Part model, mm, in its own coordinate system. Face numbers are marked on the shaded views. A direction names the side the tool comes from. Round coordinates to 2 decimals unless told otherwise and drop trailing zeros. Write each loop counter-clockwise with the first axis right and the second up, starting at its lowest first coordinate (ties: lowest second). Pieces come first, ordered by that corner, then holes. Notation, with made-up numbers: (74.25, -33.75) -> (118.25, -33.75) arc R19 ccw to (118.25, -9.75) -> close; hole circle Ø10 at (-12, 62.25). An arc over 180 degrees is marked (long way). Use CSV: the item, a comma, the result in double quotes. Start each with the question number.
(1) Drop flat-ended pins along their axis: pin 1 (6 mm diameter, centred on x = -36.5, y = 25.83, fed in from -Z); pin 2 (17.5 mm diameter, centred on y = 21, z = 88.5, fed in from +X); pin 3 (1.5 mm diameter, centred on x = -40.5, z = 2.5, fed in from +Y); pin 4 (19 mm diameter, centred on y = -11.5, z = 72.5, fed in from -X). Give the stop position or say it passes through.
(2) Saw through at C-C (y = 0). Give the cut face in (x, z).
(3) Which spindle directions (+Z, -Z, +X, -X, +Y, -Y) get a long thin tool onto all of the face, cutting with end or side? Do the marked faces 1 and 2. Say none if no direction does.
(4) Saw through at A-A (x = -48.5). Give the cut face in (y, z), plus the area to 3 significant figures.
(5) Two-plate mould, pull along Y, no slides. Class the marked faces 3, 4 and 5: released by +Y, released by -Y, zero draft, split by the parting line, or undercut.
(6) Probe line 1 (X direction, y = 17.5, z = 61.5); line 2 (Y direction, x = 2.5, z = 91.5); line 3 (X direction, y = 0, z = 104). List the from-to ranges inside material, lowest first. Write a range as [from, to].
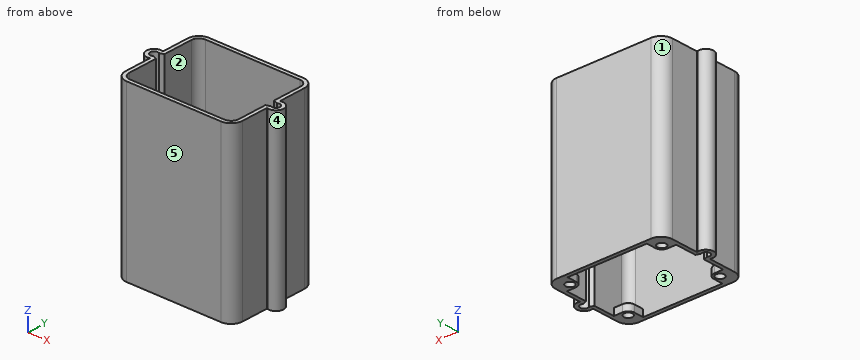
```python
from build123d import *

# Parameters (mm, degrees)
EXTRUDE_THIN1_DEPTH = 135
SKETCH6_R           = 3.429
BOSS_EXTRUDE1_DEPTH = 6
FILLET1_R           = 1


with BuildPart() as part:
    # Sketch4 → Extrude-Thin1 (new body)
    with BuildSketch(Plane.XY):
        with BuildLine():
            Line((-46.5, 27.5), (-46.5, 5.907156632))
            Line((-46.5, 5.907156632), (-46.877529279, 5.776468537))
            ThreePointArc((-46.877529279, 5.776468537), (-54.5, 0), (-46.877529279, -5.776468537))
            Line((-46.877529279, -5.776468537), (-46.5, -5.907156632))
            Line((-46.5, -5.907156632), (-46.5, -27.5))
            ThreePointArc((-46.5, -27.5), (-43.863961031, -33.863961031), (-37.5, -36.5))
            Line((-37.5, -36.5), (37.5, -36.5))
            ThreePointArc((37.5, -36.5), (43.863961031, -33.863961031), (46.5, -27.5))
            Line((46.5, -27.5), (46.5, -5.907156632))
            Line((46.5, -5.907156632), (46.877529279, -5.776468537))
            ThreePointArc((46.877529279, -5.776468537), (54.5, 0), (46.877529279, 5.776468537))
            Line((46.877529279, 5.776468537), (46.5, 5.907156632))
            Line((46.5, 5.907156632), (46.5, 27.5))
            ThreePointArc((46.5, 27.5), (43.863961031, 33.863961031), (37.5, 36.5))
            Line((37.5, 36.5), (-37.5, 36.5))
            ThreePointArc((-37.5, 36.5), (-43.863961031, 33.863961031), (-46.5, 27.5))
        make_face()
        with BuildLine():
            Line((-43.5, 27.5), (-43.5, 3.770994321))
            Line((-43.5, 3.770994321), (-46.9586126, 2.573737532))
            ThreePointArc((-46.9586126, 2.573737532), (-51.5, 0), (-46.9586126, -2.573737532))
            Line((-46.9586126, -2.573737532), (-43.5, -3.770994321))
            Line((-43.5, -3.770994321), (-43.5, -27.5))
            ThreePointArc((-43.5, -27.5), (-41.742640687, -31.742640687), (-37.5, -33.5))
            Line((-37.5, -33.5), (37.5, -33.5))
            ThreePointArc((37.5, -33.5), (41.742640687, -31.742640687), (43.5, -27.5))
            Line((43.5, -27.5), (43.5, -3.770994321))
            Line((43.5, -3.770994321), (46.9586126, -2.573737532))
            ThreePointArc((46.9586126, -2.573737532), (51.5, 0), (46.9586126, 2.573737532))
            Line((46.9586126, 2.573737532), (43.5, 3.770994321))
            Line((43.5, 3.770994321), (43.5, 27.5))
            ThreePointArc((43.5, 27.5), (41.742640687, 31.742640687), (37.5, 33.5))
            Line((37.5, 33.5), (-37.5, 33.5))
            ThreePointArc((-37.5, 33.5), (-41.742640687, 31.742640687), (-43.5, 27.5))
        make_face(mode=Mode.SUBTRACT)
    extrude(amount=EXTRUDE_THIN1_DEPTH)

    # Sketch6 → Boss-Extrude1 (add)
    with BuildSketch(Plane(origin=(0, 0, 0), x_dir=(-1, 0, 0), z_dir=(0, 0, -1))):
        with BuildLine():
            Line((-31.5, 25.830127019), (-31.5, 33.5))
            Line((-31.5, 33.5), (-37.5, 33.5))
            ThreePointArc((-37.5, 33.5), (-41.742640687, 31.742640687), (-43.5, 27.5))
            Line((-43.5, 27.5), (-43.5, 20.830127019))
            Line((-43.5, 20.830127019), (-36.5, 20.830127019))
            ThreePointArc((-36.5, 20.830127019), (-32.964466094, 22.294593113), (-31.5, 25.830127019))
        make_face()
        with Locations((-36.5, 25.830127019)):
            Circle(SKETCH6_R, mode=Mode.SUBTRACT)
        with BuildLine():
            Line((37.5, 33.5), (31.5, 33.5))
            Line((31.5, 33.5), (31.5, 25.830127019))
            ThreePointArc((31.5, 25.830127019), (32.964466094, 22.294593113), (36.5, 20.830127019))
            Line((36.5, 20.830127019), (43.5, 20.830127019))
            Line((43.5, 20.830127019), (43.5, 27.5))
            ThreePointArc((43.5, 27.5), (41.742640687, 31.742640687), (37.5, 33.5))
        make_face()
        with Locations((36.5, 25.830127019)):
            Circle(SKETCH6_R, mode=Mode.SUBTRACT)
        with BuildLine():
            Line((31.5, -25.830127019), (31.5, -33.5))
            Line((31.5, -33.5), (37.5, -33.5))
            ThreePointArc((37.5, -33.5), (41.742640687, -31.742640687), (43.5, -27.5))
            Line((43.5, -27.5), (43.5, -20.830127019))
            Line((43.5, -20.830127019), (36.5, -20.830127019))
            ThreePointArc((36.5, -20.830127019), (32.964466094, -22.294593113), (31.5, -25.830127019))
        make_face()
        with Locations((36.5, -25.830127019)):
            Circle(SKETCH6_R, mode=Mode.SUBTRACT)
        with BuildLine():
            Line((-37.5, -33.5), (-31.5, -33.5))
            Line((-31.5, -33.5), (-31.5, -25.830127019))
            ThreePointArc((-31.5, -25.830127019), (-32.964466094, -22.294593113), (-36.5, -20.830127019))
            Line((-36.5, -20.830127019), (-43.5, -20.830127019))
            Line((-43.5, -20.830127019), (-43.5, -27.5))
            ThreePointArc((-43.5, -27.5), (-41.742640687, -31.742640687), (-37.5, -33.5))
        make_face()
        with Locations((-36.5, -25.830127019)):
            Circle(SKETCH6_R, mode=Mode.SUBTRACT)
    extrude(amount=-BOSS_EXTRUDE1_DEPTH)

    # Fillet1
    fillet1_edges = [part.edges().sort_by_distance(p)[0] for p in [
        (-40, 20.830127019, 6),
        (-32.964466094, 22.294593113, 6),
        (-31.5, 29.665063509, 6),
        (-32.964466094, -22.294593113, 6),
        (-40, -20.830127019, 6),
        (-31.5, -29.665063509, 6),
        (40, -20.830127019, 6),
        (32.964466094, -22.294593113, 6),
        (31.5, -29.665063509, 6),
        (32.964466094, 22.294593113, 6),
        (40, 20.830127019, 6),
        (31.5, 29.665063509, 6),
    ]]
    fillet(fillet1_edges, radius=FILLET1_R)


solid = part.part
```
Answers:
1,pin 1,"passes through"
1,pin 2,"stops at x = 46.5"
1,pin 3,"stops at y = 36.21"
1,pin 4,"stops at x = -54.16"
2,outline,"(-54.5, 0) -> (-51.5, 0) -> (-51.5, 135) -> (-54.5, 135) -> close; (51.5, 0) -> (54.5, 0) -> (54.5, 135) -> (51.5, 135) -> close"
3,face 1,"+Z, -Z, -X, +Y"
3,face 2,"+Z"
4,outline,"(-6, 0) -> (-3, 0) -> (-3, 135) -> (-6, 135) -> close; (3, 0) -> (6, 0) -> (6, 135) -> (3, 135) -> close"
4,area,"810 mm²"
5,face 3,"undercut"
5,face 4,"split by the parting line"
5,face 5,"released by -Y"
6,line 1,"x = [-46.5, -43.5], [43.5, 46.5]"
6,line 2,"y = [-36.5, -33.5], [33.5, 36.5]"
6,line 3,"x = [-54.5, -51.5], [51.5, 54.5]"
